Build history of the part. All positions in model axes, mm. A direction names the side the tool comes from. Give positions to 0.01 mm unless a question says otherwise; leave off trailing zeros. Write each loop counter-clockwise with the first axis right and the second up, starting at its lowest first coordinate (ties: lowest second). Pieces come first, ordered by that corner, then holes. Notation, with made-up numbers: (80.5, 57.5) -> (94.5, 57.5) arc R30 cw to (94.5, 81.5) -> close; hole circle Ø9 at (-23.5, -26). An arc over 180 degrees is marked (long way). Put each result on its own line as item: value. Start each with the question number.
Item 1: Tool access for faces 1 (the flat face through (156, 3, -32)), 2 (the flat face through (80, 3, -3)), 3 (the flat face through (3, 3, -50)), 4 (the flat face through (135, 3, -72)), 5 (the flat face through (121, 3, -34)): list every direction of +Z, -Z, +X, -X, +Y, -Y with a clear straight run to the whole face (end or side of a thin tool).
Item 2: Flat gauge pins, fed straight in: pin 1 Ø3 at (x, y) = (3, 4) entering from +Z; pin 2 Ø1.5 at (y, z) = (3, -42.5) entering from +X; pin 3 Ø3 at (y, z) = (2.5, -72) entering from +X; pin 4 Ø9.5 at (x, z) = (116.5, -9) entering from +Y. Where does each tip first touch, or does it go through?
Item 3: Slice it at B-B, the plane z = -9. List the corners of the cut face in (x, y), plus the area to 3 significant figures.
Item 4: Slice it at D-D, the plane x = 12.5. List the corners of the cut face in (y, z), plus the area to 3 significant figures.
Item 5: Drill centre lines: line 1 along X through (y, z) = (2.1, -9); line 2 along X through (y, z) = (3.2, -33.5); line 3 along Z through (x, y) = (88.5, 0.45). Where is each one in solid material? Low to high.
Item 6: Two-plate mould, pull along Z, no slides. Class faces 6 (the flat face through (180, 3, -59)), 7 (the cylindrical face through (95.14, 2.96, -59.1)), 8 (the flat face through (67, 3, -69)): pulls with the +Z half, pulls with the -Z half, needs draft (parallel to the pull), parting line crosses it, or undercut.
Item 7: Slice it at C-C, the plane y = 2.9. Give the number of separate pieces and of enclosed holes in the cut face, plus the area to 3 significant figures.
Item 8: Slice it at A-A, the plane x = 116.5. List the corners of the cut face in (y, z).
```python
from build123d import *

# Parameters (mm, degrees)
SKETCH1_W           = 180
SKETCH1_H           = 75
BOSS_EXTRUDE1_DEPTH = 6
SKETCH2_W           = 23
SKETCH2_H           = 4
SKETCH2_W_2         = 24
SKETCH2_W_3         = 4
SKETCH2_H_2         = 25
CUT_EXTRUDE1_DEPTH  = 6
SKETCH3_R           = 8
SKETCH3_W           = 12
SKETCH3_H           = 6
CUT_EXTRUDE5_DEPTH  = 196.092285855
FILLET1_R           = 3
SKETCH4_W           = 44.5
SKETCH4_H           = 6
SKETCH4_W_2         = 6
SKETCH4_H_2         = 5
SKETCH4_H_3         = 16
SKETCH4_H_4         = 25
SKETCH4_W_3         = 74
SKETCH4_W_4         = 45
CUT_EXTRUDE6_DEPTH  = 196.092285855


with BuildPart() as part:
    # Sketch1 → Boss-Extrude1 (new body)
    with BuildSketch(Plane(origin=(0, 0, 0), x_dir=(1, 0, 0), z_dir=(0, 1, 0))):
        with Locations((90, 37.5)):
            Rectangle(SKETCH1_W, SKETCH1_H)
    extrude(amount=BOSS_EXTRUDE1_DEPTH)

    # Sketch2 → Cut-Extrude1 (cut)
    with BuildSketch(Plane(origin=(0, 6, 0), x_dir=(1, 0, 0), z_dir=(0, 1, 0))):
        with Locations((121.5, 32)):
            Rectangle(SKETCH2_W, SKETCH2_H)
        with Locations((168, 32)):
            Rectangle(SKETCH2_W_2, SKETCH2_H)
        with Locations((78, 37.5)):
            Rectangle(SKETCH2_W_3, SKETCH2_H_2)
    extrude(amount=-CUT_EXTRUDE1_DEPTH, mode=Mode.SUBTRACT)

    # Sketch3 → Cut-Extrude5 (cut, through all)
    with BuildSketch(Plane(origin=(0, 6, 0), x_dir=(1, 0, 0), z_dir=(0, 1, 0))):
        with Locations(Location((91, 9, 0), (0, 0, 270))):
            Circle(SKETCH3_R)
        with Locations(Location((116.5, 9, 0), (0, 0, 270))):
            Circle(SKETCH3_R)
        with Locations((90, 57)):
            Rectangle(SKETCH3_W, SKETCH3_H)
    extrude(amount=-CUT_EXTRUDE5_DEPTH, mode=Mode.SUBTRACT)

    # Fillet1
    fillet1_edges = [part.edges().sort_by_distance(p)[0] for p in [
        (96, 3, -54),
        (96, 3, -60),
        (84, 3, -54),
        (84, 3, -60),
    ]]
    fillet(fillet1_edges, radius=FILLET1_R - 0.0001)  # a hair under: the kernel refuses the full size

    # Sketch4 → Cut-Extrude6 (cut, through all)
    with BuildSketch(Plane(origin=(0, 6, 0), x_dir=(1, 0, 0), z_dir=(0, 1, 0))):
        with Locations((151.75, 3)):
            Rectangle(SKETCH4_W, SKETCH4_H)
        with Locations((177, 3)):
            Rectangle(SKETCH4_W_2, SKETCH4_H)
        with Locations((177, 27.5)):
            Rectangle(SKETCH4_W_2, SKETCH4_H_2)
        with Locations((177, 42)):
            Rectangle(SKETCH4_W_2, SKETCH4_H_3)
        with Locations((3, 37.5)):
            Rectangle(SKETCH4_W_2, SKETCH4_H_4)
        with Locations((3, 3)):
            Rectangle(SKETCH4_W_2, SKETCH4_H)
        with Locations((43, 3)):
            Rectangle(SKETCH4_W_3, SKETCH4_H)
        with Locations((157.5, 72)):
            Rectangle(SKETCH4_W_4, SKETCH4_H)
        with Locations((67.5, 72)):
            Rectangle(SKETCH4_W_4, SKETCH4_H)
    extrude(amount=-CUT_EXTRUDE6_DEPTH, mode=Mode.SUBTRACT)


solid = part.part
```
Values follow:
1. face 1: +X, +Y, -Y
1. face 2: +Z, -X, +Y, -Y
1. face 3: -X, +Y, -Y
1. face 4: -Z, +X, +Y, -Y
1. face 5: +Y, -Y
2. pin 1: z = -6
2. pin 2: x = 174
2. pin 3: x = 135
2. pin 4: through
3. outline: (0, 0) -> (83, 0) -> (83, 6) -> (0, 6) -> close; (99, 0) -> (108.5, 0) -> (108.5, 6) -> (99, 6) -> close; (124.5, 0) -> (180, 0) -> (180, 6) -> (124.5, 6) -> close
3. area: 888 mm2
4. outline: (0, -75) -> (6, -75) -> (6, -6) -> (0, -6) -> close
4. area: 414 mm2
5. line 1: 0 to 83, 99 to 108.5, 124.5 to 180
5. line 2: 6 to 76, 80 to 110, 133 to 156
5. line 3: -69 to -60, -54 to -16.6, -1.4 to 0
6. face 6: needs draft
6. face 7: undercut
6. face 8: pulls with the -Z half
7. separate pieces: 1
7. enclosed holes: 5
7. area: 11,100 mm2
8. outline: (0, -75) -> (6, -75) -> (6, -34) -> (0, -34) -> close; (0, -30) -> (6, -30) -> (6, -17) -> (0, -17) -> close; (0, -1) -> (6, -1) -> (6, 0) -> (0, 0) -> close
